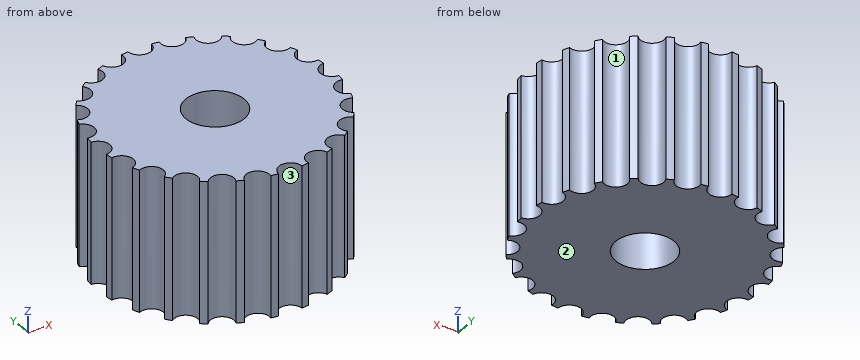
from build123d import *

# Parameters (mm, degrees)
SKETCH1_R               = 10
BOSS_EXTRUDE1_DEPTH     = 12
CUT_EXTRUDE1_DEPTH      = 19.547236991
CUT_EXTRUDE1_DEPTH_BACK = 19.547236991
SKETCH2_R               = 1
SKETCH3_R               = 2.5
CUT_EXTRUDE2_DEPTH      = 19.493377193


with BuildPart() as part:
    # Sketch1 → Boss-Extrude1 (new body)
    with BuildSketch(Plane.XY):
        Circle(SKETCH1_R)
    extrude(amount=BOSS_EXTRUDE1_DEPTH)

    # Sketch2 → Cut-Extrude1 (cut, two sides: drawn at the far end of the back side and taken through both)
    with BuildSketch(Plane.XY.offset(12).offset(-CUT_EXTRUDE1_DEPTH_BACK)):
        with Locations((0, 10)):
            Circle(SKETCH2_R)
        with Locations((2.588190451, 9.659258263)):
            Circle(SKETCH2_R)
        with Locations((5, 8.660254038)):
            Circle(SKETCH2_R)
        with Locations((7.071067812, 7.071067812)):
            Circle(SKETCH2_R)
        with Locations((8.660254038, 5)):
            Circle(SKETCH2_R)
        with Locations((9.659258263, 2.588190451)):
            Circle(SKETCH2_R)
        with Locations((10, 0)):
            Circle(SKETCH2_R)
        with Locations((9.659258263, -2.588190451)):
            Circle(SKETCH2_R)
        with Locations((8.660254038, -5)):
            Circle(SKETCH2_R)
        with Locations((7.071067812, -7.071067812)):
            Circle(SKETCH2_R)
        with Locations((5, -8.660254038)):
            Circle(SKETCH2_R)
        with Locations((2.588190451, -9.659258263)):
            Circle(SKETCH2_R)
        with Locations((0, -10)):
            Circle(SKETCH2_R)
        with Locations((-2.588190451, -9.659258263)):
            Circle(SKETCH2_R)
        with Locations((-5, -8.660254038)):
            Circle(SKETCH2_R)
        with Locations((-7.071067812, -7.071067812)):
            Circle(SKETCH2_R)
        with Locations((-8.660254038, -5)):
            Circle(SKETCH2_R)
        with Locations((-9.659258263, -2.588190451)):
            Circle(SKETCH2_R)
        with Locations((-10, 0)):
            Circle(SKETCH2_R)
        with Locations((-9.659258263, 2.588190451)):
            Circle(SKETCH2_R)
        with Locations((-8.660254038, 5)):
            Circle(SKETCH2_R)
        with Locations((-7.071067812, 7.071067812)):
            Circle(SKETCH2_R)
        with Locations((-5, 8.660254038)):
            Circle(SKETCH2_R)
        with Locations((-2.588190451, 9.659258263)):
            Circle(SKETCH2_R)
    extrude(amount=CUT_EXTRUDE1_DEPTH + CUT_EXTRUDE1_DEPTH_BACK, mode=Mode.SUBTRACT)

    # Sketch3 → Cut-Extrude2 (cut, through all)
    with BuildSketch(Plane.XY.offset(12)):
        Circle(SKETCH3_R)
    extrude(amount=-CUT_EXTRUDE2_DEPTH, mode=Mode.SUBTRACT)


solid = part.part
For this review, take the finished solid that the model builds, in its own axes (mm). Face numbers are marked on the shaded views. Coordinates: 2 decimals unless noted, no trailing zeros. Loops run counter-clockwise (first coordinate to the right, second up) from the corner with the lowest first, then second, coordinate; pieces in that order, holes last. Notation, with made-up numbers: (-38.75, 3.25) - (-27.75, 3.25) arc R16 ccw to (-27.75, 9.25) - close; hole circle Ø10 at (43.5, 4.25). An arc over 180 degrees is marked (long way). Use a Markdown table: item, result. Add a question column.
Item 1: We need section D-D (y = -5). Give the boundary of the cut face in (x, z), and give its area (3 significant figures).
Item 2: Mouldability with a two-part tool opening along Y and no side actions: class the marked faces 1, 2 and 3 as pulls with the +Y half, pulls with the -Y half, needs draft (parallel to the pull), parting line crosses it, or undercut.
Item 3: We need section A-A (x = 0). Give the boundary of the cut face in (y, z).
Item 4: We need section C-C (x = 7.25). Give the boundary of the cut face in (y, z).
Item 5: For line 1 (X direction, y = 0.25, z = 10.5); line 2 (Y direction, x = 0.75, z = 4.75); line 3 (X direction, y = 2.25, z = 3.5), list the stretches that pass through material, from the lowest coordinate up.
Item 6: Insertion check: pin 1 Ø1.5 at (x, z) = (5, 2.5) entering from -Y; pin 2 Ø5 at (x, z) = (4, 2) entering from +Y; pin 3 Ø5 at (x, z) = (-6, 8.5) entering from +Y. Each pin has a flat end and moves straight along its axis. Give the tip position at first contact, or say it passes through.
Results list:
| question | item | result |
|---|---|---|
| 1 | outline | (-7.66, 0) - (7.66, 0) - (7.66, 12) - (-7.66, 12) - close |
| 1 | area | 184 mm^2 |
| 2 | face 1 | undercut |
| 2 | face 2 | needs draft |
| 2 | face 3 | pulls with the -Y half |
| 3 | outline | (-9, 0) - (-2.5, 0) - (-2.5, 12) - (-9, 12) - close; (2.5, 0) - (9, 0) - (9, 12) - (2.5, 12) - close |
| 4 | outline | (-6.09, 0) - (6.09, 0) - (6.09, 12) - (-6.09, 12) - close |
| 5 | line 1 | x = -9.03 to -2.49, 2.49 to 9.03 |
| 5 | line 2 | y = -9.34 to -2.38, 2.38 to 9.34 |
| 5 | line 3 | x = -8.72 to -1.09, 1.09 to 8.72 |
| 6 | pin 1 | stops at y = -8 |
| 6 | pin 2 | stops at y = 9.89 |
| 6 | pin 3 | stops at y = 9.35 |
